Print and shaded views of the part. All mm, measured from the part's lowest x, y and z. A direction names the side the tool comes from. Give positions to 0.01 mm unless a question says otherwise; leave off trailing zeros. Loops run counter-clockwise (first coordinate to the right, second up) from the corner with the lowest first, then second, coordinate; pieces in that order, holes last. Notation, with made-up numbers: (6, 27.25) -> (59, 27.25) arc R16 ccw to (59, 58.25) -> close; hole circle Ø9 at (15, 33). An arc over 180 degrees is marked (long way). Answer as a JSON object with one key per item and string values. Group by question number.
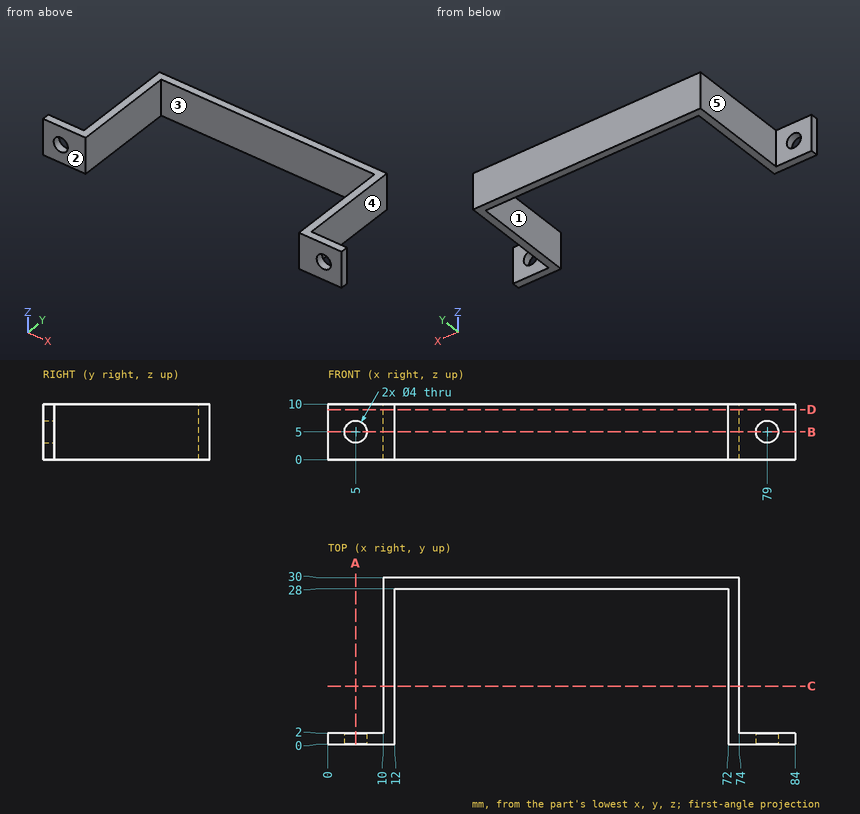
(1) Pull direction X, two halves, no side cores. Call the marked faces 3, 4 and 5: pulls with the +X half, pulls with the -X half, needs draft (parallel to the pull), parting line crosses it, or undercut.
(2) Saw through at C-C on y = 10.5. List the corners of the cut face in (x, z).
(3) Saw through at A-A on x = 5. List the corners of the cut face in (y, z).
(4) 3-axis set-ups, long thin cutter, end or side, ignore diameter. For the marked faces 1 and 2: which of +Z, -Z, +X, -X, +Y, -Y reach the whole face in a straight line?
(5) Saw through at D-D on z = 9. List the corners of the cut face in (x, y), plus the area to 3 significant figures.
(6) Saw through at B-B on z = 5. List the corners of the cut face in (x, y), plus the area to 3 significant figures.
(7) Probe line 1 along X through (y, z) = (0.5, 5); line 2 along X through (y, z) = (17.25, 5); line 3 along Z through (x, y) = (5, 1.6). List the from-to ranges inside material, lowest first. Write a range as [from, to].
(8) Pin check, flat tips, straight feed: pin 1 (3 mm diameter, centred on y = 13, z = 6.5, fed in from -X); pin 2 (4 mm diameter, centred on y = 7.5, z = 3.5, fed in from +X); pin 3 (1 mm diameter, centred on x = 12, z = 4, fed in from -Y); pin 4 (3 mm diameter, centred on x = 53.5, z = 5, fed in from -Y). Stop position of each tip, or through.
Calculated:
{
 "1": {"face 3": "undercut", "face 4": "pulls with the +X half", "face 5": "pulls with the -X half"},
 "2": {"outline": "(10, 0) -> (12, 0) -> (12, 10) -> (10, 10) -> close; (72, 0) -> (74, 0) -> (74, 10) -> (72, 10) -> close"},
 "3": {"outline": "(0, 0) -> (2, 0) -> (2, 3) -> (0, 3) -> close; (0, 7) -> (2, 7) -> (2, 10) -> (0, 10) -> close"},
 "4": {"face 1": "+Z, -Z, -Y", "face 2": "+Z, -Z, +X, -X, -Y"},
 "5": {"outline": "(0, 0) -> (12, 0) -> (12, 28) -> (72, 28) -> (72, 0) -> (84, 0) -> (84, 2) -> (74, 2) -> (74, 30) -> (10, 30) -> (10, 2) -> (0, 2) -> close", "area": "280 mm^2"},
 "6": {"outline": "(0, 0) -> (3, 0) -> (3, 2) -> (0, 2) -> close; (7, 0) -> (12, 0) -> (12, 28) -> (72, 28) -> (72, 0) -> (77, 0) -> (77, 2) -> (74, 2) -> (74, 30) -> (10, 30) -> (10, 2) -> (7, 2) -> close; (81, 0) -> (84, 0) -> (84, 2) -> (81, 2) -> close", "area": "264 mm^2"},
 "7": {"line 1": "x = [0, 3], [7, 12], [72, 77], [81, 84]", "line 2": "x = [10, 12], [72, 74]", "line 3": "z = [0, 3], [7, 10]"},
 "8": {"pin 1": "stops at x = 10", "pin 2": "stops at x = 74", "pin 3": "stops at y = 0", "pin 4": "stops at y = 28"}
}
